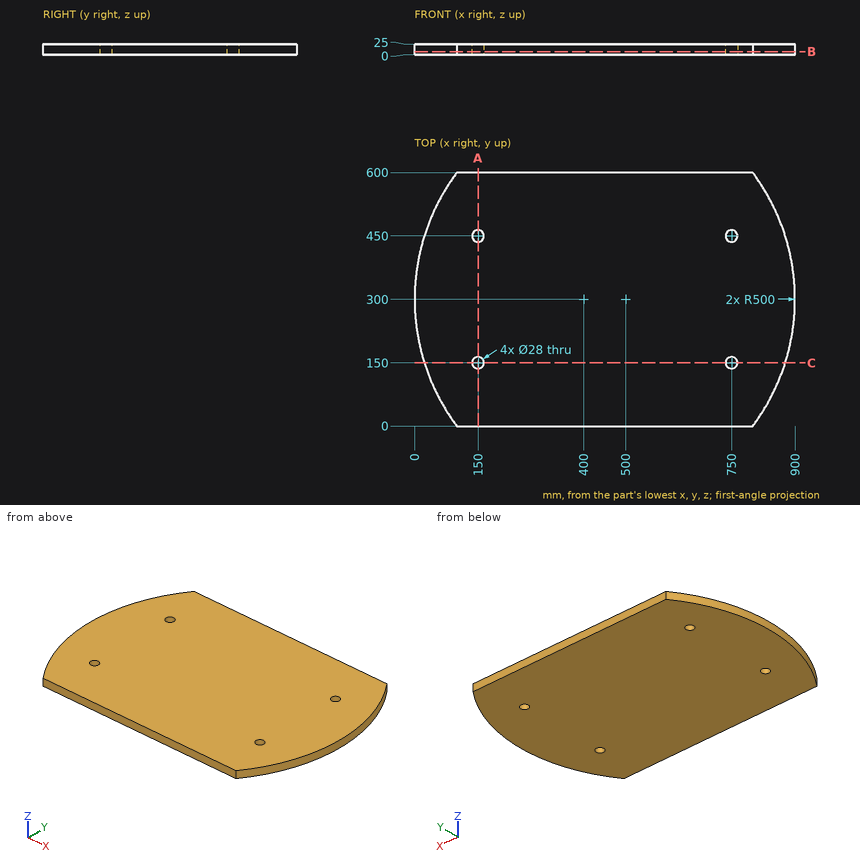
Job drawing, mm, ordinate dimensions from the low corner. One solid piece. Coordinates: 2 decimals unless noted, no trailing zeros. Write each loop counter-clockwise with the first axis right and the second up, starting at its lowest first coordinate (ties: lowest second). Pieces come first, ordered by that corner, then holes. Notation, with made-up numbers: (48, -36) -> (107, -36) arc R15 ccw to (107, -30) -> close; hole circle Ø1 at (45, 30.25). An arc over 180 degrees is marked (long way). Use CSV: the item, a comma, the result in double quotes. Start each with the question number.
Item 1: Wall check: probe 1 along Y at (x, z) = (750, 16); probe 2 along Y at (x, z) = (744, 7.25); probe 3 along Y at (x, z) = (850.5, 23.25). Give the ranges that are in metal, low to high.
Item 2: Band-saw the part on C-C, the plane y = 150. Write the cut outline in (x, z), plus the area to 3 significant figures.
Item 3: Band-saw the part on B-B, the plane z = 7. Write the cut outline in (x, y).
Item 4: Drop flat-ended pins along their axis: P1, Ø5, axis at y = 514, z = 20.5, coming from the +X side; P2, Ø25, axis at x = 150, y = 150, coming from the +Z side; P3, Ø10, axis at y = 469, z = 8, coming from the +X side. Give the stop position or say it passes through.
Item 5: Band-saw the part on A-A, the plane x = 150. Write the cut outline in (y, z), plus the area to 3 significant figures.
Response values:
1,probe 1,"y = 0 to 136, 164 to 436, 464 to 600"
1,probe 2,"y = 0 to 137.35, 162.65 to 437.35, 462.65 to 600"
1,probe 3,"y = 83.09 to 516.91"
2,outline,"(23.03, 0) -> (136, 0) -> (136, 25) -> (23.03, 25) -> close; (164, 0) -> (736, 0) -> (736, 25) -> (164, 25) -> close; (764, 0) -> (876.97, 0) -> (876.97, 25) -> (764, 25) -> close"
2,area,"19,900 mm2"
3,outline,"(100, 0) -> (800, 0) arc R500 ccw to (800, 600) -> (100, 600) arc R500 ccw to start; hole circle Ø28 at (150, 150); hole circle Ø28 at (150, 450); hole circle Ø28 at (750, 150); hole circle Ø28 at (750, 450)"
4,P1,"stops at x = 853.06"
4,P2,"passes through"
4,P3,"stops at x = 872.34"
5,outline,"(0, 0) -> (136, 0) -> (136, 25) -> (0, 25) -> close; (164, 0) -> (436, 0) -> (436, 25) -> (164, 25) -> close; (464, 0) -> (600, 0) -> (600, 25) -> (464, 25) -> close"
5,area,"13,600 mm2"
